Autodesk Inventor part; units mm, degrees
ref_plane "Start Plane" through (0, 0, 20) normal (0, 0, 1) x (1, 0, 0)
ref_plane "End Plane" through (0, 0, 365) normal (0, 0, 1) x (1, 0, 0)
ref_plane "Work Plane4" through (162.5, -7, 365) normal (0, 0, 1) x (1, 0, 0)
ref_plane "Start Plane" through (0, 0, 20) normal (0, 0, 1) x (1, 0, 0)
ref_plane "End Plane" through (0, 0, 365) normal (0, 0, 1) x (1, 0, 0)
sketch "Sketch" plane through (0, 0, 0) normal (0, 0, 1) x (1, 0, 0)
  line L0 (-10, -7) -> (-10, 7)
  line L1 (-7, 10) -> (7, 10)
  line L2 (10, 7) -> (10, -7)
  line L3 (7, -10) -> (-7, -10)
  arc A0 (-10, -7) -> (-7, -10) centre (-7, -7) ccw
  arc A1 (-7, 10) -> (-10, 7) centre (-7, 7) ccw
  arc A2 (10, 7) -> (7, 10) centre (7, 7) ccw
  arc A3 (7, -10) -> (10, -7) centre (7, -7) ccw
  line L4 (-6, 8) -> (6, 8)
  line L5 (8, 6) -> (8, -6)
  line L6 (6, -8) -> (-6, -8)
  line L7 (-8, -6) -> (-8, 6)
  line L8 (0, 14.8698) -> (0, -14.8698) construction
  line L9 (-14.8698, 0) -> (14.8698, 0) construction
  arc A4 (-8, -6) -> (-6, -8) centre (-6, -6) ccw
  arc A5 (-6, 8) -> (-8, 6) centre (-6, 6) ccw
  arc A6 (8, 6) -> (6, 8) centre (6, 6) ccw
  arc A7 (6, -8) -> (8, -6) centre (6, -6) ccw
  dimension "d7" = 3
  dimension "d10" = 20
  dimension "d11" = 20
  dimension "d12" = 2
  dimension "d15" = 10
  dimension "d16" = 10
  dimension "d19" = 2
  dimension "d20" = 2
extrude "Body" add sketch "Sketch" along normal up to surface (345 mm away) from surface at 20
sketch "Sketch3" plane through (0, 0, 0) normal (0, 0, 1) x (1, 0, 0)
  line L0 (0, 0) -> (10, 0)
ref_plane "Work Plane3" through (0, 0, 0) normal (0, -1, 0) x (1, 0, 0)
ref_plane "Work Plane4" through (162.5, -7, 365) normal (0, 0, 1) x (1, 0, 0)
split "Split1" plane through (162.5, -7, 365) removes the side toward (0, 0, 1)
ref_plane "Work Plane5" through (-162.5, -7, 20) normal (0, 0, -1) x (-1, 0, 0)
split "Split2" plane through (-162.5, -7, 20) removes the side toward (0, 0, -1)
sketch "Sketch4" plane through (0, 0, 0) normal (0, -1, 0) x (1, 0, 0)
  line L0 (-2, 20) -> (12, 20)
  line L1 (-2, 365) -> (12, 365)
  dimension "d18" = 345
equation "\"d7\" = G_IR"
equation "\"d10\" = G_H"
equation "\"d11\" = G_W"
equation "\"d12\" = G_T"
equation "\"d15\" = 0.5 * d10"
equation "\"d16\" = 0.5 * d11"
equation "\"d19\" = G_T"
equation "\"d20\" = G_T"
equation "\"d3\" = G_L"
equation "\"G_W\" = 20"
equation "\"G_H\" = 20"
equation "\"G_T\" = 2"
equation "\"G_IR\" = 3"
equation "\"G_L\" = d18"
equation "\"d14\" = G_OFFSET_END + B_L"
equation "\"B_L\" = 385"
properties part number "DIN EN 10210-2 - 20 x 20 x 2 - 345" material "Steel, Mild"
Check sheet for the modelled part. Datum: model origin and axes. Units: mm. A direction names the side the tool comes from. Round coordinates to 2 decimals unless told otherwise and drop trailing zeros. Write each loop counter-clockwise with the first axis right and the second up, starting at its lowest first coordinate (ties: lowest second). Pieces come first, ordered by that corner, then holes. Notation, with made-up numbers: M -14,6.5 L 43,6.5 A31 cw 43,41.5 Z; hole C 33.25,-7 d2. An arc over 180 degrees is marked long. Write item = value, one per line. Start each with the question number.
1. Section check C-C, the plane z = 294. Record the cut outline in (x, y), then the cut area to 3 significant figures.
2. Scan lines: line 1 (Y direction, x = 1.75, z = 85.5); line 2 (X direction, y = -6.5, z = 243.5); line 3 (X direction, y = 6.25, z = 117.5). Record each from-to range of solid material in increasing order. Write a range as [from, to].
3. Release check for a two-part mould opening along X. For faces 3 (the flat face through (0, -10, 190)), 4 (the flat face through (-8, 0, 190)), 5 (the flat face through (-10, 0, 190)) record: pulls with the +X half, pulls with the -X half, needs draft (parallel to the pull), parting line crosses it, or undercut.
4. Tool access check on faces 1 (the flat face through (8, 0, 190)), 2 (the flat face through (0, 10, 190)). Record the directions out of +Z, -Z, +X, -X, +Y, -Y that give a thin tool (end or side, any length) a straight path to the whole face; none if there is none.
5. Section check A-A, the plane y = -3. Record the cut outline in (x, z).
Results found:
q1.outline = M -10,-7 A3 ccw -7,-10 L 7,-10 A3 ccw 10,-7 L 10,7 A3 ccw 7,10 L -7,10 A3 ccw -10,7 Z; hole M -8,-6 A2 ccw -6,-8 L 6,-8 A2 ccw 8,-6 L 8,6 A2 ccw 6,8 L -6,8 A2 ccw -8,6 Z
q1.area = 140 mm^2
q2.line_1 = [-10, -8], [8, 10]
q2.line_2 = [-10, -7.94], [7.94, 10]
q2.line_3 = [-10, -7.98], [7.98, 10]
q3.face_3 = needs draft
q3.face_4 = undercut
q3.face_5 = pulls with the -X half
q4.face_1 = +Z, -Z
q4.face_2 = +Z, -Z, +X, -X, +Y
q5.outline = M -10,20 L -8,20 L -8,365 L -10,365 Z; M 8,20 L 10,20 L 10,365 L 8,365 Z
